Model file for the job. Use its own axes, mm. A direction names the side the tool comes from. Round coordinates to 2 decimals unless told otherwise and drop trailing zeros. Loops run counter-clockwise (first coordinate to the right, second up) from the corner with the lowest first, then second, coordinate; pieces in that order, holes last. Notation, with made-up numbers: M 62.25,63 L 76.25,63 A24 cw 76.25,79 Z; hole C -31,19.25 d5. An arc over 180 degrees is marked long. Use a Markdown table: item, result. Add a question column.
Item 1: Two-plate mould, pull along X, no slides. Class faces 1 (the flat face through (31, -11, 10)), 2 (the cylindrical face through (0.66, 29.993, 9.86)), 3 (the flat face through (1.9, 30.1, 20)): +X half, -X half, draft (parallel to the pull), parting line (faces both ways), or undercut.
Item 2: Pin check, flat tips, straight feed: P1, Ø10, axis at y = -6.5, z = 17, coming from the -X side; P2, Ø10, axis at y = 10, z = 3, coming from the +X side; P3, Ø6, axis at y = -18, z = 12, coming from the +X side. Stop position of each tip, or through.
Item 3: Saw through at C-C on z = 9.5. Write the cut outline in (x, y).
Item 4: Saw through at A-A on y = -1. Write the cut outline in (x, z).
Item 5: Wall check: L1, parallel to X at y = -24.6, z = 10; L2, parallel to X at y = -2, z = 5.25; L3, parallel to X at y = -24.55, z = 10. Give the ranges that are in metal, low to high. Write a range as from..to.
Item 6: Saw through at D-D on z = 13.75. Write the cut outline in (x, y), then the cut area to 3 significant figures.
Item 7: Tool access for faces 4 (the flat face through (43, -25, 10)), 5 (the flat face through (43, -24, 10)), 6 (the flat face through (-36, -25.8, 10)), 7 (the cylindrical face through (30.68, -24.35, 9.86)): list every direction of +Z, -Z, +X, -X, +Y, -Y with a clear straight run to the whole face (end or side of a thin tool).
Item 8: Saw through at B-B on x = 40. Write the cut outline in (y, z).
```python
from build123d import *

# Parameters (mm, degrees)
BASE_FLANGE1_DEPTH = 20
SKETCH6_R          = 2.5
CUT_EXTRUDE1_DEPTH = 10
FILLET1_R          = 0.5


# Sheet-metal steps are written as plain solids
with BuildPart() as part:
    # Sketch1 → Base-Flange1 (new body)
    with BuildSketch(Plane.XY):
        with BuildLine():
            Line((50, -25), (32.27, -25))
            ThreePointArc((32.27, -25), (30.664867607, -24.335132393), (30, -22.73))
            Line((30, -22.73), (30, 0))
            ThreePointArc((30, 0), (0, 30), (-30, 0))
            Line((-30, 0), (-30, -24.53))
            ThreePointArc((-30, -24.53), (-30.664867607, -26.135132393), (-32.27, -26.8))
            Line((-32.27, -26.8), (-40, -26.8))
            Line((-40, -26.8), (-40, -25.8))
            Line((-40, -25.8), (-32.27, -25.8))
            ThreePointArc((-32.27, -25.8), (-31.371974388, -25.428025612), (-31, -24.53))
            Line((-31, -24.53), (-31, 0))
            ThreePointArc((-31, 0), (0, 31), (31, 0))
            Line((31, 0), (31, -22.73))
            ThreePointArc((31, -22.73), (31.371974388, -23.628025612), (32.27, -24))
            Line((32.27, -24), (50, -24))
            Line((50, -24), (50, -25))
        make_face()
    extrude(amount=BASE_FLANGE1_DEPTH)

    # Sketch6 → Cut-Extrude1 (cut)
    with BuildSketch(Plane(origin=(0, -24, 0), x_dir=(1, 0, 0), z_dir=(0, 1, 0))):
        with Locations(Location((40, -10, 0), (0, 0, 270))):
            Circle(SKETCH6_R)
    extrude(amount=-CUT_EXTRUDE1_DEPTH, mode=Mode.SUBTRACT)

    # Fillet1
    fillet1_edges = [part.edges().sort_by_distance(p)[0] for p in [
        (50, -24.5, 0),
        (-40, -26.3, 0),
        (50, -24.5, 20),
        (-40, -26.3, 20),
    ]]
    fillet(fillet1_edges, radius=FILLET1_R)


solid = part.part
```
Entries:
| question | item | result |
|---|---|---|
| 1 | face 1 | +X half |
| 1 | face 2 | undercut |
| 1 | face 3 | draft |
| 2 | P1 | x = -31 |
| 2 | P2 | x = 30.59 |
| 2 | P3 | x = 31 |
| 3 | outline | M -40,-26.8 L -32.27,-26.8 A2.27 ccw -30,-24.53 L -30,0 A30 cw 30,0 L 30,-22.73 A2.27 ccw 32.27,-25 L 37.55,-25 L 37.55,-24 L 32.27,-24 A1.27 cw 31,-22.73 L 31,0 A31 ccw -31,0 L -31,-24.53 A1.27 cw -32.27,-25.8 L -40,-25.8 Z; M 42.45,-25 L 50,-25 L 50,-24 L 42.45,-24 Z |
| 4 | outline | M -31,0 L -30,0 L -30,20 L -31,20 Z; M 30,0 L 31,0 L 31,20 L 30,20 Z |
| 5 | L1 | -31..-30, 30.98..37.5, 42.5..50 |
| 5 | L2 | -31..-30, 30..31 |
| 5 | L3 | -31..-30, 30.91..37.5, 42.5..50 |
| 6 | outline | M -40,-26.8 L -32.27,-26.8 A2.27 ccw -30,-24.53 L -30,0 A30 cw 30,0 L 30,-22.73 A2.27 ccw 32.27,-25 L 50,-25 L 50,-24 L 32.27,-24 A1.27 cw 31,-22.73 L 31,0 A31 ccw -31,0 L -31,-24.53 A1.27 cw -32.27,-25.8 L -40,-25.8 Z |
| 6 | area | 174 mm2 |
| 7 | face 4 | +Z, -Z, +X, -Y |
| 7 | face 5 | +Z, -Z, +X, +Y |
| 7 | face 6 | +Z, -Z, -X, +Y |
| 7 | face 7 | +Z, -Z, -Y |
| 8 | outline | M -25,0 L -24,0 L -24,7.5 L -25,7.5 Z; M -25,12.5 L -24,12.5 L -24,20 L -25,20 Z |
